Source: three-view drawing plus pictorial views. Frame: mm from the lowest corner of the part. A direction names the side the tool comes from. Coordinates: 2 decimals unless noted, no trailing zeros. Order: outer loops, then holes, each group sorted by start corner. A loop starts at its lowest first (then second) coordinate and runs counter-clockwise, first axis right, second up. Notation, with made-up numbers: (76, -21) -> (122, -21) arc R22 cw to (122, -14) -> close; hole circle Ø11 at (-33, -25). An arc over 180 degrees is marked (long way). Use one line per item in the form item = value. Start each with the question number.
1) Draft query along Y for the marked faces 3, 4 and 5. Return one class per face: pulls with the +Y half, pulls with the -Y half, needs draft (parallel to the pull), parting line crosses it, or undercut.
2) Section query D-D on y = 13.75. Output: boundary loops of the cut face in (x, z), then the cut area to 3 significant figures.
3) Section query A-A on y = 7.5. Output: boundary loops of the cut face in (x, z).
4) Access query for the marked faces 1 and 2. Directions: +Z, -Z, +X, -X, +Y, -Y. A direction counts if a zero-diameter tool reaches every point of the face in a straight line with its end or side. Return the directions, or none.
5) Section query C-C on z = 16.5. Output: boundary loops of the cut face in (x, y).
6) Ray query, line 1 along X through (y, z) = (4, 16.5); line 2 along Z through (x, y) = (10.25, 6.25); line 3 along Y through (x, z) = (13.75, 6.5). Return the intervals inside material, ascending.
7) Section query B-B on x = 16. Output: boundary loops of the cut face in (y, z), then the cut area to 3 significant figures.
8) Pin query (flat end, axial travel): pin 1 (6.5 mm diameter, centred on y = 9.5, z = 13.5, fed in from +X); pin 2 (5 mm diameter, centred on x = 12, y = 10, fed in from +Z); pin 3 (6 mm diameter, centred on x = 10, y = 11, fed in from -Z). Return the tip coordinate at first contact, or that it passes through.
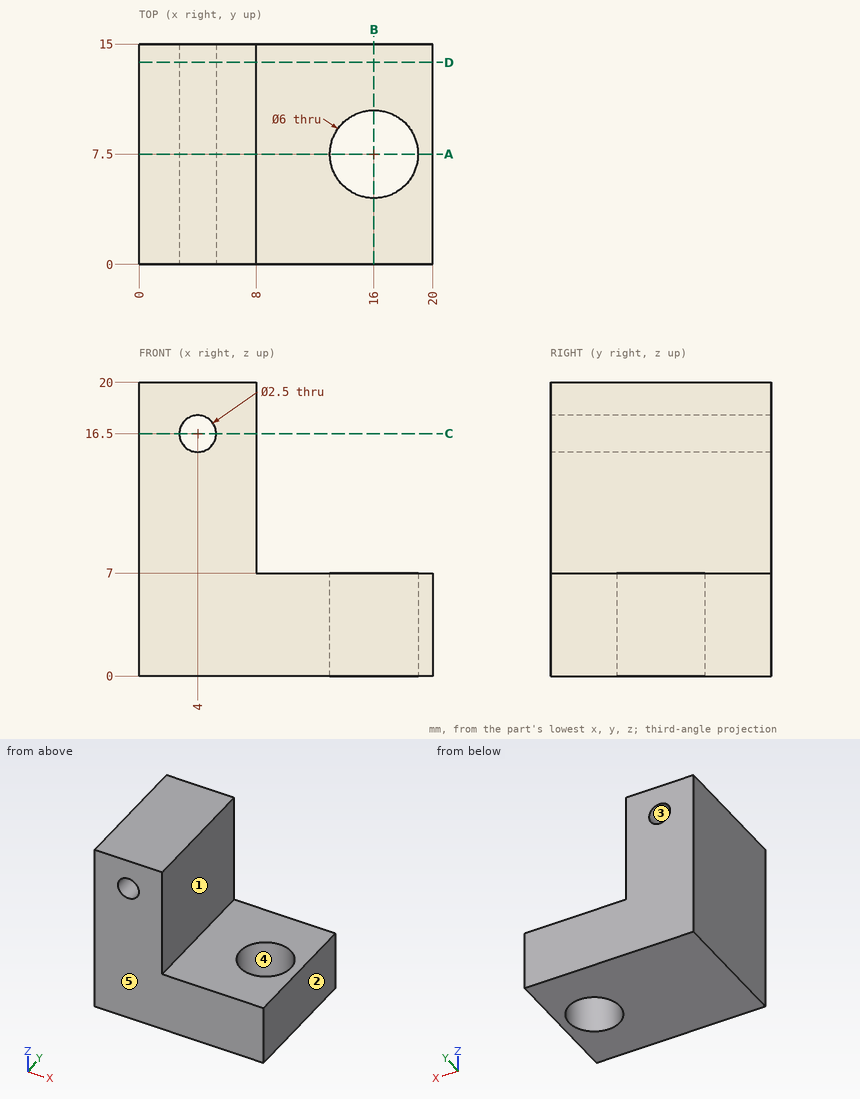
Answers below:
q1.face_3 = needs draft
q1.face_4 = undercut
q1.face_5 = pulls with the -Y half
q2.outline = (0, 0) -> (20, 0) -> (20, 7) -> (8, 7) -> (8, 20) -> (0, 20) -> close; hole circle Ø2.5 at (4, 16.5)
q2.area = 239 mm^2
q3.outline = (0, 0) -> (13, 0) -> (13, 7) -> (8, 7) -> (8, 20) -> (0, 20) -> close; (19, 0) -> (20, 0) -> (20, 7) -> (19, 7) -> close; hole circle Ø2.5 at (4, 16.5)
q4.face_1 = +Z, +X, +Y, -Y
q4.face_2 = +Z, -Z, +X, +Y, -Y
q5.outline = (0, 0) -> (2.75, 0) -> (2.75, 15) -> (0, 15) -> close; (5.25, 0) -> (8, 0) -> (8, 15) -> (5.25, 15) -> close
q6.line_1 = 0 to 2.75, 5.25 to 8
q6.line_2 = 0 to 7
q6.line_3 = 0 to 5.52, 9.48 to 15
q7.outline = (0, 0) -> (4.5, 0) -> (4.5, 7) -> (0, 7) -> close; (10.5, 0) -> (15, 0) -> (15, 7) -> (10.5, 7) -> close
q7.area = 63.0 mm^2
q8.pin_1 = 8
q8.pin_2 = 7
q8.pin_3 = 0
